For this review, take the finished solid that the model builds, in its own axes (mm). Coordinates: 2 decimals unless noted, no trailing zeros. Write each loop counter-clockwise with the first axis right and the second up, starting at its lowest first coordinate (ties: lowest second). Pieces come first, ordered by that corner, then holes. Notation, with made-up numbers: M 67,-38 L 125,-38 A21 cw 125,-4 Z; hole C 65.25,11.5 d11. An arc over 180 degrees is marked long. Return JSON: item names as keys, results as strings.
```python
from build123d import *

# Parameters (mm, degrees)
SKETCH1_W                    = 90
SKETCH1_H                    = 40
BOSS_EXTRUDE1_DEPTH          = 8
SKETCH2_R                    = 16
CUT_EXTRUDE1_DEPTH           = 61.737138556
F_7_0_7_DIAMETER_HOLE1_D     = 7
F_7_0_7_DIAMETER_HOLE1_DEPTH = 60
F_7_0_7_DIAMETER_HOLE1_TIP   = 2.103012167
M4X0_7_TAPPED_HOLE1_D        = 3.3
CHAMFER1_SIZE                = 2


with BuildPart() as part:
    # Sketch1 → Boss-Extrude1 (new body)
    with BuildSketch(Plane(origin=(0, 0, 0), x_dir=(0, 0, -1), z_dir=(1, 0, 0))):
        with Locations((0, 20)):
            Rectangle(SKETCH1_W, SKETCH1_H)
    extrude(amount=BOSS_EXTRUDE1_DEPTH)

    # Sketch2 → Cut-Extrude1 (cut, through all)
    with BuildSketch(Plane(origin=(8, 0, 0), x_dir=(0, 0, -1), z_dir=(1, 0, 0))):
        with Locations((0, 20)):
            Circle(SKETCH2_R)
    extrude(amount=-CUT_EXTRUDE1_DEPTH, mode=Mode.SUBTRACT)

    # Ø7.0 (7) Diameter Hole1
    with Locations(Plane(origin=(8, 0, 0), x_dir=(0, 0, -1), z_dir=(1, 0, 0))):
        with Locations((-39, 6), (39, 6), (39, 34), (-39, 34)):
            Hole(F_7_0_7_DIAMETER_HOLE1_D / 2, depth=F_7_0_7_DIAMETER_HOLE1_DEPTH)
            with Locations((0, 0, -(F_7_0_7_DIAMETER_HOLE1_DEPTH + F_7_0_7_DIAMETER_HOLE1_TIP / 2))):  # 118° drill point
                Cone(0, F_7_0_7_DIAMETER_HOLE1_D / 2, F_7_0_7_DIAMETER_HOLE1_TIP, mode=Mode.SUBTRACT)

    # M4x0.7 Tapped Hole1 (through all)
    with Locations(Plane(origin=(8, 0, 0), x_dir=(0, 0, -1), z_dir=(1, 0, 0))):
        with Locations((16.263455967, 36.263455967), (-16.263455967, 3.736544033)):
            Hole(M4X0_7_TAPPED_HOLE1_D / 2)

    # Chamfer1
    chamfer1_edges = [part.edges().sort_by_distance(p)[0] for p in [
        (4, 0, -45),
        (4, 0, 45),
        (4, 40, 45),
        (4, 40, -45),
    ]]
    chamfer(chamfer1_edges, length=CHAMFER1_SIZE)


solid = part.part
```
1. We need section D-D (y = 25.5). State the section outline as (x, z) points, plus the area to 3 significant figures.
Checks:
{"outline": "M 0,-45 L 8,-45 L 8,-15.02 L 0,-15.02 Z; M 0,15.02 L 8,15.02 L 8,45 L 0,45 Z", "area": "480 mm2"}
2. We need section C-C (z = 39). State the section outline as (x, y) points, plus the area to 3 significant figures.
Checks:
{"outline": "M 0,0 L 8,0 L 8,2.5 L 0,2.5 Z; M 0,9.5 L 8,9.5 L 8,30.5 L 0,30.5 Z; M 0,37.5 L 8,37.5 L 8,40 L 0,40 Z", "area": "208 mm2"}
3. We need section B-B (y = 8). State the section outline as (x, z) points, plus the area to 3 significant figures.
Checks:
{"outline": "M 0,-45 L 8,-45 L 8,-41.87 L 0,-41.87 Z; M 0,-36.13 L 8,-36.13 L 8,-10.58 L 0,-10.58 Z; M 0,10.58 L 8,10.58 L 8,36.13 L 0,36.13 Z; M 0,41.87 L 8,41.87 L 8,45 L 0,45 Z", "area": "459 mm2"}
4. Clearance check with a flat-ended pin moving along its axis: pin 1 Ø4 at (y, z) = (33, -2) entering from +X. State where the tip first meets the part, or that it passes through.
Checks:
{"pin 1": "through"}
5. Draft analysis for pull direction Z (two halves, no side actions). For faces 1 (the face through (4, 39, 44)), 2 (the face through (4.06, 4.38, 3.47)), 3 (the face through (4, 20, -45)), state which applies: +Z half, -Z half, draft (parallel to the pull), parting line (faces both ways), or undercut.
Checks:
{"face 1": "+Z half", "face 2": "undercut", "face 3": "-Z half"}
6. Wall thickness on L1, parallel to Y at x = 5.5, z = 39; L2, parallel to Z at x = 2.5, y = 8; L3, parallel to Z at x = 4.5, y = 17: over which ranges is each line inside the solid? List them lowest first. Write a range as from..to.
Checks:
{"L1": "0..2.5, 9.5..30.5, 37.5..40", "L2": "-45..-41.87, -36.13..-10.58, 10.58..36.13, 41.87..45", "L3": "-45..-15.72, 15.72..45"}
7. We need section A-A (z = 0). State the section outline as (x, y) points.
Checks:
{"outline": "M 0,0 L 8,0 L 8,4 L 0,4 Z; M 0,36 L 8,36 L 8,40 L 0,40 Z"}
